Verification items for the finished model (mm, model axes). Face numbers are marked on the shaded views. A direction names the side the tool comes from. Round coordinates to 2 decimals unless told otherwise and drop trailing zeros. Order: outer loops, then holes, each group sorted by start corner. A loop starts at its lowest first (then second) coordinate and runs counter-clockwise, first axis right, second up. Notation, with made-up numbers: (-37, -33.75) -> (9, -33.75) arc R7 ccw to (9, -21.75) -> close; hole circle Ø10 at (-22, 52). An arc over 180 degrees is marked (long way). Put each result on its own line as item: value.
Autodesk Fusion 360 part; units mm, degrees
sketch "Sketch1" plane through (0, 0, 0) normal (0, 1, 0) x (1, 0, 0)
  line L0 (0, 0) -> (12.4, 0)
  line L1 (12.4, 0) -> (12.4, -25.75)
  line L2 (12.4, -25.75) -> (0, -25.75)
  line L3 (0, -25.75) -> (0, 0)
  line L4 (0, 0) -> (-5.3, 0)
  line L5 (-5.3, 0) -> (-5.3, -25.75)
  line L6 (-5.3, -25.75) -> (0, -25.75)
  line L7 (0, -25.75) -> (0, 0)
  line L8 (12.4, 0) -> (17.7, 0)
  line L9 (17.7, 0) -> (17.7, -25.75)
  line L10 (17.7, -25.75) -> (12.4, -25.75)
  line L11 (12.4, -25.75) -> (12.4, 0)
  line L12 (-5.3, -25.75) -> (-2.675, -25.75)
  line L13 (-2.675, -25.75) -> (-2.675, -23.25)
  line L14 (-2.675, -23.25) -> (-5.3, -23.25)
  line L15 (-5.3, -23.25) -> (-5.3, -25.75)
  line L16 (-2.675, -23.25) -> (15.075, -23.25)
  line L17 (-2.675, -23.25) -> (-2.675, -2.5)
  circle A0 centre (-2.675, -23.25) radius 1.25
  circle A1 centre (-2.675, -2.5) radius 1.25
  circle A2 centre (15.075, -23.25) radius 1.25
  line L18 (-2.675, -2.5) -> (15.075, -2.5)
  circle A3 centre (15.075, -2.5) radius 1.25
  dimension "d1" = 12.4
  dimension "d2" = 25.75
  dimension "d3" = 5.3
  dimension "d4" = 5.3
  dimension "d5" = 25.75
  dimension "d6" = 25.75
  dimension "d13" = 2.625
  dimension "d14" = 2.5
  dimension "d15" = 17.75
  dimension "d16" = 20.75
  dimension "d17" = 2.5
  dimension "d18" = 2.5
  dimension "d19" = 2.5
  dimension "d20" = 17.75
  dimension "d21" = 2.5
extrude "Extrude1" add sketch "Sketch1" along normal blind 5.3 contours L0 L1 L3 L7 L11 L18 | L3 L4 L5 L7 L14 L17 A0 A1 L18 | A3 | A2 | L1 L8 L9 L10 L11 | L1 L3 L7 L11 L16 L18 | L3 L7 L16 L17 A0 A1 L18 | L1 L2 L3 L7 L11 L16 | L3 L6 L7 L13 L16 A0 | L17 A1 L18 | L17 A1 L18 | L5 L6 L12 L13 L14 L15 A0 | L13 L16 A0 | L16 L17 A0 | L14 L17 A0 | L13 L14 A0
extrude "Extrude2" add sketch "Sketch1" along normal blind 20 contours L3 L4 L5 L7 L14 L17 A0 A1 L18 | A3 | A2 | L1 L8 L9 L10 L11 | L3 L7 L16 L17 A0 A1 L18 | L3 L6 L7 L13 L16 A0 | L17 A1 L18 | L17 A1 L18 | L5 L6 L12 L13 L14 L15 A0 | L13 L16 A0 | L16 L17 A0 | L14 L17 A0 | L13 L14 A0
extrude "Extrude3" cut sketch "Sketch1" along normal up to surface (20 mm away) contours A3 | A2 | L17 A1 L18 | L17 A1 L18 | L13 L16 A0 | L16 L17 A0 | L14 L17 A0 | L13 L14 A0
sketch "Sketch3" plane through (0, 20, 0) normal (0, 1, 0) x (-1, 0, 0)
  circle A0 centre (2.675, 23.25) radius 1.25
  circle A1 centre (2.675, 2.5) radius 1.25
  line L0 (0, 25.75) -> (0, 0)
  line L1 (0, 0) -> (5.3, 0)
  line L2 (5.3, 0) -> (5.3, 25.75)
  line L3 (5.3, 25.75) -> (0, 25.75)
  line L4 (2.675, 2.5) -> (2.675, 5)
  line L5 (2.675, 5) -> (0, 5)
  line L6 (2.675, 5) -> (5.3, 5)
  line L7 (2.675, 23.25) -> (2.675, 20.75)
  line L8 (2.675, 20.75) -> (-2, 20.75)
  line L9 (-2, 20.75) -> (2.675, 20.75)
  line L10 (7.8916, 20.75) -> (2.675, 20.75)
  dimension "d24" = 2.5
  dimension "d25" = 2.5
extrude "Extrude4" cut sketch "Sketch3" against normal blind 14.7 contours L0 L2 L3 L8 L9 L10 | L0 L1 L2 L5 L6
sketch "Sketch4" plane through (0, 20, 0) normal (0, 1, 0) x (-1, 0, 0)
  circle A0 centre (-15.075, 23.25) radius 1.25
  circle A1 centre (-15.075, 2.5) radius 1.25
  line L0 (-12.4, 25.75) -> (-17.7, 25.75)
  line L1 (-17.7, 25.75) -> (-17.7, 0)
  line L2 (-17.7, 0) -> (-12.4, 0)
  line L3 (-12.4, 0) -> (-12.4, 25.75)
  line L4 (-15.075, 2.5) -> (-15.075, 5)
  line L5 (-9.6971, 5) -> (-24, 5)
  line L6 (-15.075, 23.25) -> (-15.075, 20.75)
  line L7 (-20.719, 20.75) -> (-5, 20.75)
  dimension "d28" = 2.5
  dimension "d29" = 2.5
extrude "Extrude5" cut sketch "Sketch4" against normal blind 14.7 contours L0 L1 L3 L7 | L1 L2 L3 L5
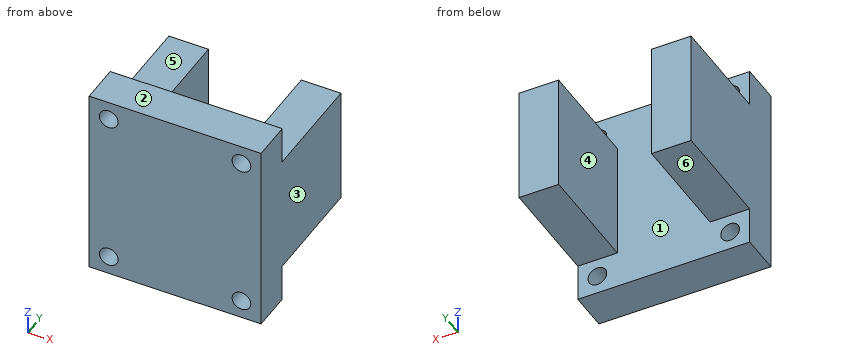
Item 1: Release check for a two-part mould opening along X. For the marked faces 1, 2 and 3 record: pulls with the +X half, pulls with the -X half, needs draft (parallel to the pull), parting line crosses it, or undercut.
Geometry check:
face 1: undercut
face 2: needs draft
face 3: pulls with the +X half
Item 2: Depth check by flat-ended pin: pin 1 Ø3 at (x, y) = (-1.5, 11.5) entering from -Z; pin 2 Ø3 at (x, z) = (-2.675, 2.5) entering from +Y; pin 3 Ø1.6 at (x, y) = (15.5, 9.5) entering from +Z. Enter the tip coordinate at first touch or a pass-through.
Geometry check:
pin 1: z = 5
pin 2: y = 5.3
pin 3: z = 20.75
Item 3: Sectioned sample at A-A, the plane y = 1.5. Record the boundary of the cut face in (x, z) (3 decimals), then the cut area to 3 significant figures.
Geometry check:
outline: (-5.3, 0) -> (17.7, 0) -> (17.7, 25.75) -> (-5.3, 25.75) -> close; hole circle Ø2.5 at (-2.675, 2.5); hole circle Ø2.5 at (-2.675, 23.25); hole circle Ø2.5 at (15.075, 2.5); hole circle Ø2.5 at (15.075, 23.25)
area: 573 mm2
Item 4: Sectioned sample at D-D, the plane z = 18.25. Record the boundary of the cut face in (x, y).
Geometry check:
outline: (-5.3, 0) -> (17.7, 0) -> (17.7, 20) -> (12.4, 20) -> (12.4, 5.3) -> (0, 5.3) -> (0, 20) -> (-5.3, 20) -> close
Item 5: Material ranges on line 1 along X through (y, z) = (2.05, 23.25) (3 decimals); line 2 along X through (y, z) = (8.5, 17.5); line 3 along Y through (x, z) = (7.5, 20), recorded low to high.
Geometry check:
line 1: -5.3 to -3.925, -1.425 to 13.825, 16.325 to 17.7
line 2: -5.3 to 0, 12.4 to 17.7
line 3: 0 to 5.3
Item 6: Tool access check on the marked faces 4, 5 and 6. Record the directions out of +Z, -Z, +X, -X, +Y, -Y that give a thin tool (end or side, any length) a straight path to the whole face; none if there is none.
Geometry check:
face 4: +Z, -Z, +Y
face 5: +Z, +X, -X, +Y
face 6: -Z, +X, -X, +Y
Item 7: Sectioned sample at C-C, the plane y = 17. Record the boundary of the cut face in (x, z).
Geometry check:
outline: (-5.3, 5) -> (0, 5) -> (0, 20.75) -> (-5.3, 20.75) -> close; (12.4, 5) -> (17.7, 5) -> (17.7, 20.75) -> (12.4, 20.75) -> close
Item 8: Sectioned sample at B-B, the plane z = 23.25. Record the boundary of the cut face in (x, y) (3 decimals).
Geometry check:
outline: (-5.3, 0) -> (-3.925, 0) -> (-3.925, 5.3) -> (-5.3, 5.3) -> close; (-1.425, 0) -> (13.825, 0) -> (13.825, 5.3) -> (-1.425, 5.3) -> close; (16.325, 0) -> (17.7, 0) -> (17.7, 5.3) -> (16.325, 5.3) -> close
